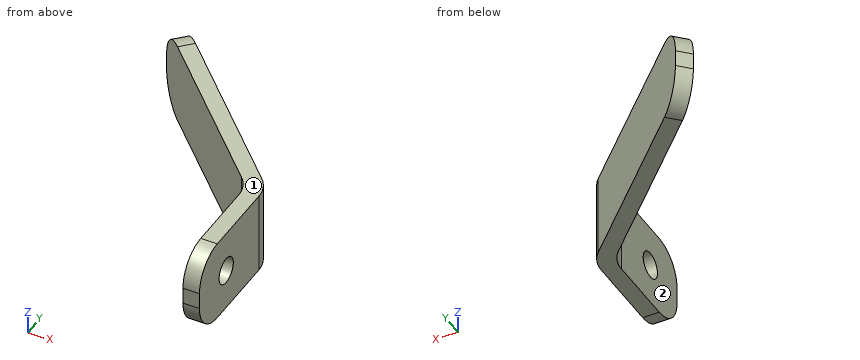
Autodesk Inventor part; units mm, degrees
ref_plane "YZ Plane" through (0, 0, 0) normal (1, 0, 0) x (0, 1, 0)
ref_plane "XZ Plane" through (0, 0, 0) normal (0, 1, 0) x (-1, 0, 0)
ref_plane "XY Plane" through (0, 0, 0) normal (0, 0, 1) x (1, 0, 0)
ref_plane "Arbeitsebene1" through (0, 0, 0) normal (0, 0, 1) x (1, 0, 0)
sketch "Skizze1" plane through (0, 0, 0) normal (0, 0, 1) x (1, 0, 0)
  line L0 (0, 10.5) -> (-10, 10.5)
  line L1 (0, 13.3) -> (-10, 13.3)
  line L2 (-10.5, 0) -> (-10.5, 117.8)
  line L3 (-10.5, 4.5) -> (-12.5, 4.5)
  line L4 (-12.5, 4.5) -> (-12.5, 19.5)
  line L5 (-12.5, 19.5) -> (-10.5, 19.5)
  line L6 (-10.5, 19.5) -> (-10.5, 4.5)
  line L7 (-10.5, 19.5) -> (-31.7883, 40.6378)
  line L8 (-31.7883, 40.6378) -> (-33.1975, 39.2186)
  line L9 (-33.1975, 39.2186) -> (-12.5, 18.6674)
  line L10 (-29.2442, 38.1116) -> (-8.6029, 58.9) construction
  line L11 (2, 58.9) -> (-12, 58.9)
  point P0 (0, 0)
  point P1 (-10.5, 19.5)
  dimension "d0" = 2
  dimension "d1" = 15
  dimension "d2" = 6
  dimension "d3" = 2
  dimension "d4" = 30
  dimension "d5" = 90
extrude "Extrusion1" add sketch "Skizze1" along normal blind 10
fillet "Rundung1" radius 4 6 edges at (-12.5, 18.6674, 5) (-10.5, 19.5, 5) (-11.5, 4.5, 10) (-11.5, 4.5, 0) (-32.4929, 39.9282, 10) (-32.4929, 39.9282, 0)
sketch "Skizze2" plane through (-12.5, 8.5, 0) normal (-1, 0, 0) x (0, 0, 1)
  arc A0 (0, 0) -> (4, -4) centre (4, 0) ccw
  line L0 (4, -4) -> (6, -4)
  arc A1 (6, -4) -> (10, 0) centre (6, 0) ccw
  line L1 (10, 8.5022) -> (10, 0)
  line L2 (0, 8.5022) -> (10, 8.5022)
  line L3 (0, 8.5022) -> (0, 0)
  circle A2 centre (5, 2) radius 1.6
  point P0 (0, -8.5)
  dimension "d9" = 3.2
  dimension "d10" = 6
extrude "Extrusion2" cut sketch "Skizze2" against normal blind 10 contours A2
properties part number "30_Cameraholder"
Check sheet for the modelled part. Datum: model origin and axes. Units: mm. Face numbers are marked on the shaded views. A direction names the side the tool comes from. Coordinates: 2 decimals unless noted, no trailing zeros. Order: outer loops, then holes, each group sorted by start corner. A loop starts at its lowest first (then second) coordinate and runs counter-clockwise, first axis right, second up. Notation, with made-up numbers: M -38.75,51 L 5.25,51 A29 cw 5.25,76 Z; hole C 8.5,27 d8. An arc over 180 degrees is marked long. Write each question's results on one line, items separated by ' | '. Start each with the question number.
1. Material ranges on probe 1 along X at (y, z) = (15, 6.5); probe 2 along Y at (x, z) = (-11.6, 5); probe 3 along Y at (x, z) = (-11.15, 5), recorded low to high.
2. Access from +Z, -Z, +X, -X, +Y, -Y to the whole of each face (thin tool, end or side, straight path). Record for the marked faces 1 and 2.
3. Go/stop test with flat-tipped pins: P1, Ø12, axis at x = -31, y = 21, coming from the +Z side; P2, Ø3, axis at y = 36.5, z = 8, coming from the -X side; P3, Ø4, axis at x = -22, z = 8.5, coming from the +Y side; P4, Ø5, axis at y = 12.5, z = 2.5, coming from the -X side. Record where each tip stops, or that it passes through.
4. Cross-section at A-A on y = 10.5. Record the cut outline in (x, z).
5. Cross-section at B-B on z = 5. Record the cut outline in (x, y).
6. Cross-section at C-C on z = 0.5. Record the cut outline in (x, y).
7. Cross-section at D-D on x = -15. Record the cut outline in (y, z), and give its area (3 significant figures).
Checks:
1) probe 1: x = -12.5 to -10.5 | probe 2: y = 4.5 to 8.9, 12.1 to 20.59 | probe 3: y = 4.5 to 8.9, 12.1 to 20.02
2) face 1: +Z, +X, -X, +Y, -Y | face 2: +Z, -Z, -X, -Y
3) P1: passes through | P2: stops at x = -31.97 | P3: stops at y = 32.9 | P4: stops at x = -12.5
4) outline: M -12.5,0 L -10.5,0 L -10.5,3.4 L -12.5,3.4 Z; M -12.5,6.6 L -10.5,6.6 L -10.5,10 L -12.5,10 Z
5) outline: M -33.2,39.22 L -13.68,19.84 A4 cw -12.5,17 L -12.5,12.1 L -10.5,12.1 L -10.5,17.83 A4 ccw -11.68,20.67 L -31.79,40.64 Z; M -12.5,4.5 L -10.5,4.5 L -10.5,8.9 L -12.5,8.9 Z
6) outline: M -31.73,37.76 L -13.68,19.84 A4 cw -12.5,17 L -12.5,6.56 L -10.5,6.56 L -10.5,17.83 A4 ccw -11.68,20.67 L -30.32,39.18 Z
7) outline: M 21.15,0 L 23.97,0 L 23.97,10 L 21.15,10 Z | area: 28.2 mm²
